Autodesk Inventor part; units mm, degrees
ref_plane "YZ Plane" through (0, 0, 0) normal (1, 0, 0) x (0, 1, 0)
ref_plane "XZ Plane" through (0, 0, 0) normal (0, 1, 0) x (-1, 0, 0)
ref_plane "XY Plane" through (0, 0, 0) normal (0, 0, 1) x (1, 0, 0)
sketch "Skizze1" plane through (0, 0, 0) normal (0, 0, 1) x (1, 0, 0)
  circle A0 centre (0, 0) radius 13.75
  circle A1 centre (0, 0) radius 5
  line L0 (2.75, 2.75) -> (-2.75, 2.75)
  line L1 (-2.75, 2.75) -> (-2.75, -2.75)
  line L2 (-2.75, -2.75) -> (2.75, -2.75)
  line L3 (2.75, -2.75) -> (2.75, 2.75)
  line L4 (2.75, 2.75) -> (-2.75, -2.75) construction
  line L5 (-2.75, 2.75) -> (2.75, -2.75) construction
  line L6 (0, 13.75) -> (0, -13.75) construction
  circle A2 centre (0, 9) radius 4
  circle A3 centre (0, 9) radius 2.25
  circle A4 centre (0, -9) radius 4
  circle A5 centre (0, -9) radius 2.25
  line L7 (-13.75, 0) -> (13.75, 0) construction
  circle A6 centre (0, 0) radius 2
  dimension "d0" = 27.5
  dimension "d1" = 10
  dimension "d25" = 5.5
  dimension "d28" = 8
  dimension "d29" = 18
  dimension "d30" = 4.5
  dimension "d43" = 4
extrude "Extrusion1" add sketch "Skizze1" against normal blind 5 contours A0 | A1 | A4 | A2 | L3 L2 L1 L0
extrude "Extrusion8" cut sketch "Skizze1" against normal blind 3 contours A4 | A2
extrude "Extrusion9" add sketch "Skizze1" along normal blind 26 contours A1
extrude "Extrusion12" add sketch "Skizze1" along normal blind 3.5 contours L3 L2 L1 L0
properties part number "Schalter_Basis"
Could you check a few things on this model? Use its own coordinates, in mm. A direction names the side the tool comes from. Give positions to 0.01 mm unless a question says otherwise; leave off trailing zeros. Loops run counter-clockwise (first coordinate to the right, second up) from the corner with the lowest first, then second, coordinate; pieces in that order, holes last. Notation, with made-up numbers: (60, 68.5) - (100, 68.5) arc R26 cw to (100, 82.5) - close; hole circle Ø7 at (-34.5, -40). An arc over 180 degrees is marked (long way). Use one line per item in the form item = value.
1. I want a section at D-D (z = -2.5). Please give me the cut outline in (x, y).
Response values:
outline = circle Ø27.5 at (0, 0); hole circle Ø8 at (0, -9); hole circle Ø8 at (0, 9); hole circle Ø4 at (0, 0)
2. I need wall thicknesses on probe 1 along Y at (x, z) = (0, -0.95); probe 2 along Y at (x, z) = (0, -3.8); probe 3 along Y at (x, z) = (0, 1.25). Which ranges of each line are inside material? Lowest first, please.
Response values:
probe_1 = -13.75 to -13, -5 to -2, 2 to 5, 13 to 13.75
probe_2 = -13.75 to -11.25, -6.75 to -2, 2 to 6.75, 11.25 to 13.75
probe_3 = -5 to -2, 2 to 5
3. I want a section at B-B (x = -1.5). Give the number of separate pieces and of enclosed holes in the cut face, and give its area (3 significant figures).
Response values:
separate_pieces = 4
enclosed_holes = 0
area = 181 mm²
4. Thinking about a two-plate mould opening in X: for faces 1 (the face through (-2, 1, 3.5)), 2 (the face through (-2.981, -13.423, -2.465)), 3 (the face through (6, 0, 0)), which applies, released by +X, released by -X, zero draft, split by the parting line, or undercut?
Response values:
face_1 = undercut
face_2 = split by the parting line
face_3 = zero draft
5. I want a section at C-C (z = 20). Please give me the cut outline in (x, y), and give its area (3 significant figures).
Response values:
outline = circle Ø10 at (0, 0); hole (-2.75, -2.75) - (2.75, -2.75) - (2.75, 2.75) - (-2.75, 2.75) - close
area = 48.3 mm²
6. On a 3-axis mill with a long thin cutter (end or side, diameter ignored), from which of +Z, -Z, +X, -X, +Y, -Y can I reach the whole of each face in a straight line? I mean faces 4 (the face through (2, 7, -3)), 5 (the face through (0, -3, -5)). Say none if no direction works.
Response values:
face_4 = +Z
face_5 = -Z, +X, -X, +Y, -Y
7. I want a section at A-A (y = 0). Please give me the cut outline in (x, z), and give its area (3 significant figures).
Response values:
outline = (-13.75, -5) - (-2, -5) - (-2, 3.5) - (-2.75, 3.5) - (-2.75, 26) - (-5, 26) - (-5, 0) - (-13.75, 0) - close; (2, -5) - (13.75, -5) - (13.75, 0) - (5, 0) - (5, 26) - (2.75, 26) - (2.75, 3.5) - (2, 3.5) - close
area = 240 mm²
8. I'm going to push flat-ended pins straight in: pin 1 Ø4.5 at (y, z) = (-1, 14.5) entering from +X; pin 2 Ø6 at (x, z) = (-0.5, 19) entering from -Y; pin 3 Ø6 at (y, z) = (7.5, 1.5) entering from +X; pin 4 Ø10 at (x, y) = (3.5, -6) entering from +Z. Where does each tip first touch, or does it pass through?
Response values:
pin_1 = 5
pin_2 = -5
pin_3 = 12.85
pin_4 = 26
